Can you work these out from the model? Positions are in its coordinate system, mm. Face numbers are marked on the shaded views. A direction names the side the tool comes from. Coordinates: 2 decimals unless noted, no trailing zeros. Loops run counter-clockwise (first coordinate to the right, second up) from the corner with the lowest first, then second, coordinate; pieces in that order, holes last.
```python
from build123d import *

# Parameters (mm, degrees)
F0_W      = 80
F0_H      = 85
F1_DEPTH  = 25.4
F2_W      = 35
F2_H      = 22
F3_DEPTH  = 37.5
F4_W      = 80
F4_H      = 85
F5_DEPTH  = 12.7
F6_R      = 3.1623
F7_DEPTH  = 6.35
F8_R      = 5.08
F9_R      = 5.08
F10_R     = 5.08
F11_R     = 5.08
F12_R     = 1.27
F13_DEPTH = 2.54
F15_DEPTH = 25.4
F16_R     = 6.35
F16_R_2   = 3.81
F17_DEPTH = 6.35


with BuildPart() as f1:
    # F0 (on Top) → F1 (new body)
    with BuildSketch(Plane.XY):
        Rectangle(F0_W, F0_H)
    extrude(amount=F1_DEPTH)

    # F2 (on Front) → F3 (cut, symmetric)
    with BuildSketch(Plane.XZ):
        with Locations((0, 12.7)):
            Rectangle(F2_W, F2_H)
    extrude(amount=F3_DEPTH, both=True, mode=Mode.SUBTRACT)

    # F4 (on face) → F5 (cut)
    with BuildSketch(Plane.XY.offset(25.4)):
        Rectangle(F4_W, F4_H)
    extrude(amount=-F5_DEPTH, mode=Mode.SUBTRACT)

    # F6 (on face) → F7 (cut)
    with BuildSketch(Plane.XY.offset(12.7)):
        with Locations((-29.21, -31.75)):
            Circle(F6_R)
        with Locations((29.21, -31.75)):
            Circle(F6_R)
        with Locations((29.21, 31.75)):
            Circle(F6_R)
        with Locations((-29.21, 31.75)):
            Circle(F6_R)
    extrude(amount=-F7_DEPTH, mode=Mode.SUBTRACT)

    # F8
    f8_edges = [f1.edges().sort_by_distance(p)[0] for p in [
        (0, -42.5, 0),
    ]]
    fillet(f8_edges, radius=F8_R)

    # F9
    f9_edges = [f1.edges().sort_by_distance(p)[0] for p in [
        (40, 2.54, 0),
    ]]
    fillet(f9_edges, radius=F9_R)

    # F10
    f10_edges = [f1.edges().sort_by_distance(p)[0] for p in [
        (-2.54, 42.5, 0),
    ]]
    fillet(f10_edges, radius=F10_R)

    # F11
    f11_edges = [f1.edges().sort_by_distance(p)[0] for p in [
        (-40, 0, 0),
    ]]
    fillet(f11_edges, radius=F11_R)

    # F12 (on face) → F13 (cut)
    with BuildSketch(Plane(origin=(0, 0, 0), x_dir=(1, 0, 0), z_dir=(0, 0, -1))):
        with Locations((-21.31, 26.67)):
            Circle(F12_R)
        with Locations((-21.31, -26.67)):
            Circle(F12_R)
        with Locations((21.31, 26.67)):
            Circle(F12_R)
        with Locations((21.31, -26.67)):
            Circle(F12_R)
    extrude(amount=-F13_DEPTH, mode=Mode.SUBTRACT)

    # F14 (on face) → F15 (cut)
    with BuildSketch(Plane.XY.offset(12.7)):
        Polygon((-40, 27.7749088), (-40, -27.7749088), (-33.2500008, -23.9649088), (-33.2500008, 23.9649088), align=None)
        Polygon((33.2500008, -23.9649088), (40, -27.7749088), (40, 27.7749088), (33.2500008, 23.9649088), align=None)
    extrude(amount=-F15_DEPTH, mode=Mode.SUBTRACT)

    # F16 (on face) → F17 (cut)
    with BuildSketch(Plane.XY.offset(12.7)):
        with Locations((-29.21, -31.75)):
            Circle(F16_R)
        with Locations((-29.21, -31.75)):
            Circle(F16_R_2, mode=Mode.SUBTRACT)
        with Locations((29.21, -31.75)):
            Circle(F16_R)
        with Locations((29.21, -31.75)):
            Circle(F16_R_2, mode=Mode.SUBTRACT)
        with Locations((29.21, 31.75)):
            Circle(F16_R)
        with Locations((29.21, 31.75)):
            Circle(F16_R_2, mode=Mode.SUBTRACT)
        with Locations((-29.21, 31.75)):
            Circle(F16_R)
        with Locations((-29.21, 31.75)):
            Circle(F16_R_2, mode=Mode.SUBTRACT)
    extrude(amount=-F17_DEPTH, mode=Mode.SUBTRACT)


solid = f1.part
```
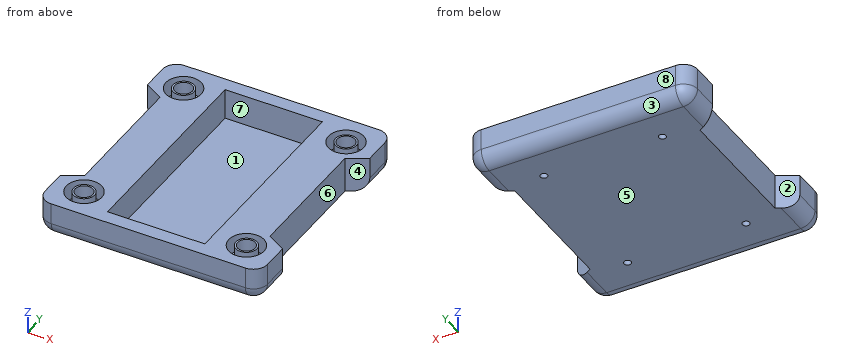
Item 1: On a 3-axis mill with a long thin cutter (end or side, diameter ignored), from which of +Z, -Z, +X, -X, +Y, -Y can I reach the whole of each face in a straight line? I mean the marked faces 1, 2, 3, 4 and 5. Say none if no direction works.
Results are:
face 1: +Z
face 2: +Z, -Z, -X
face 3: -Z, +X, -X, +Y
face 4: +Z, -Z, +X
face 5: -Z, +X, -X, +Y, -Y
Item 2: I'm going to push flat-ended pins straight in: P1, Ø3.5, axis at y = 9, z = 7.5, coming from the -X side; P2, Ø10.5, axis at x = -6.5, y = -15, coming from the +Z side; P3, Ø1, axis at y = 9.5, z = 11, coming from the +X side. Where does each tip first touch, or does it pass through?
Results are:
P1: stops at x = -33.25
P2: stops at z = 1.7
P3: stops at x = 33.25
Item 3: Suppose I cut it at C-C, the plane x = -11.5. Please give me the cut outline in (y, z).
Results are:
outline: (-42.5, 5.08) arc R5.08 ccw to (-37.42, 0) - (37.42, 0) arc R5.08 ccw to (42.5, 5.08) - (42.5, 12.7) - (37.5, 12.7) - (37.5, 1.7) - (-37.5, 1.7) - (-37.5, 12.7) - (-42.5, 12.7) - close
Item 4: I need wall thicknesses on line 1 along X through (y, z) = (19.5, 4); line 2 along Y through (x, z) = (-21.31, 0.9); line 3 along Y through (x, z) = (21.31, 1.4). Which ranges of each line are inside material? Lowest first, please.
Results are:
line 1: x = -33.25 to -17.5, 17.5 to 33.25
line 2: y = -40.31 to -27.94, -25.4 to 25.4, 27.94 to 40.31
line 3: y = -40.92 to -27.94, -25.4 to 25.4, 27.94 to 40.92
Item 5: Suppose I cut it at A-A, the plane z = 9.75. Count the separate pieces of the cut face and the enclosed holes in it, plus the area to 3 significant figures.
Results are:
separate pieces: 5
enclosed holes: 9
area: 3,000 mm2
Item 6: We'd pull the mould along X, two halves only. Please class the marked faces 6, 7 and 8: +X half, -X half, draft (parallel to the pull), parting line (faces both ways), or undercut.
Results are:
face 6: +X half
face 7: undercut
face 8: draft
Item 7: Suppose I cut it at D-D, the plane z = 3.75. Please give me the cut outline in (x, y), plus the area to 3 significant figures.
Results are:
outline: (-39.82, -37.42) arc R4.9 ccw to (-34.92, -42.32) - (34.92, -42.32) arc R4.9 ccw to (39.82, -37.42) - (39.82, -27.67) - (33.25, -23.96) - (33.25, 23.96) - (39.82, 27.67) - (39.82, 37.42) arc R4.9 ccw to (34.92, 42.32) - (-34.92, 42.32) arc R4.9 ccw to (-39.82, 37.42) - (-39.82, 27.67) - (-33.25, 23.96) - (-33.25, -23.96) - (-39.82, -27.67) - close; hole (-17.5, -37.5) - (17.5, -37.5) - (17.5, 37.5) - (-17.5, 37.5) - close
area: 3,420 mm2
